For this review, use the dimensioned drawing (mm, ordinates from the lowest corner) and the shaded views. A direction names the side the tool comes from. Coordinates: 2 decimals unless noted, no trailing zeros. Write each loop counter-clockwise with the first axis right and the second up, starting at its lowest first coordinate (ties: lowest second). Pieces come first, ordered by that corner, then holes. Notation, with made-up numbers: (77.5, 28.25) - (99.5, 28.25) arc R17 ccw to (99.5, 43.25) - close; hole circle Ø5 at (39.25, 75). An arc over 180 degrees is marked (long way). One line per item, written item: value.
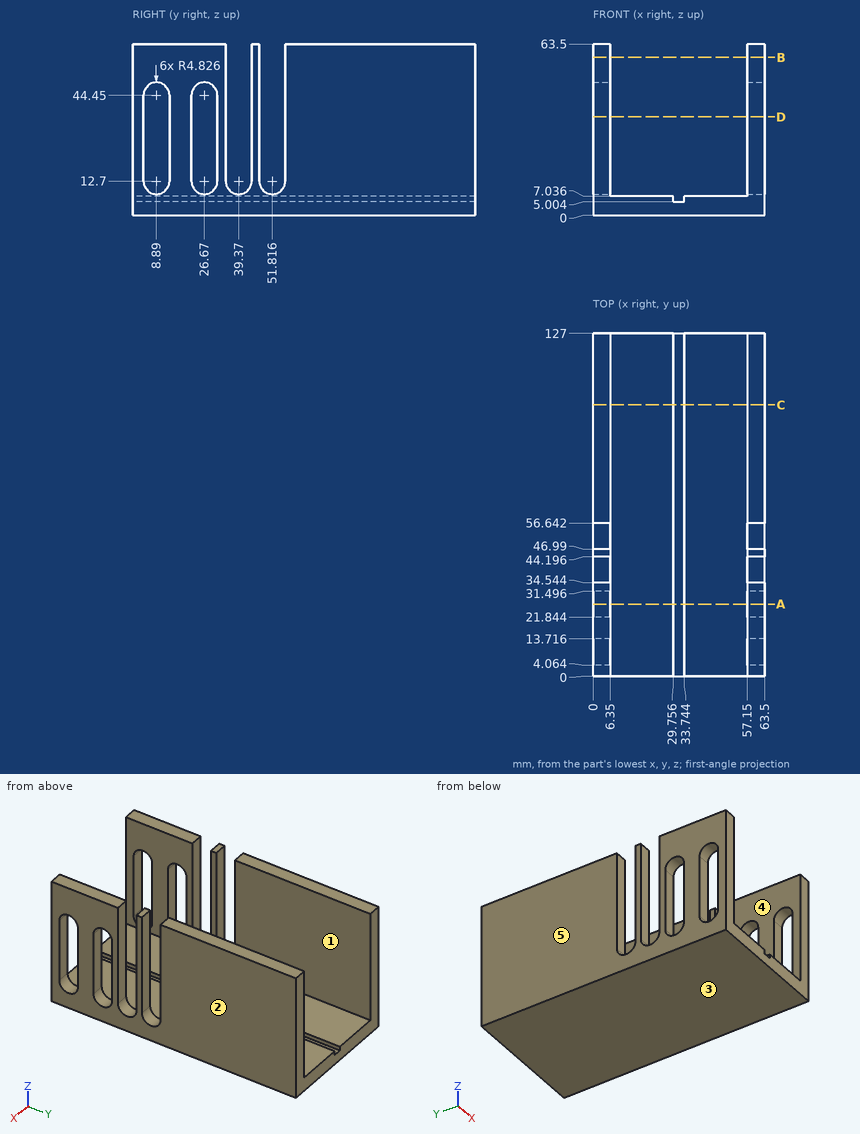
1. Consider section C-C, the plane y = 100.5. Write out the cut boundary in (x, z), then the cut area to 3 significant figures.
Answer block:
outline: (0, 0) - (63.5, 0) - (63.5, 63.5) - (57.15, 63.5) - (57.15, 7.04) - (33.74, 7.04) - (33.74, 5) - (29.76, 5) - (29.76, 7.04) - (6.35, 7.04) - (6.35, 63.5) - (0, 63.5) - close
area: 1,160 mm^2
2. Mouldability with a two-part tool opening along X and no side actions: class the marked faces 1, 2 and 3 as released by +X, released by -X, zero draft, split by the parting line, or undercut.
Answer block:
face 1: undercut
face 2: released by +X
face 3: zero draft
3. Insertion check: pin 1 Ø5 at (x, y) = (23.5, 37) entering from +Z. The pin has a flat end and moves straight along its axis. Give the tip position at first contact, or say it passes through.
Answer block:
pin 1: stops at z = 7.04
4. Consider section B-B, the plane z = 58.5. Write out the cut boundary in (x, y), then the cut area to 3 significant figures.
Answer block:
outline: (0, 0) - (6.35, 0) - (6.35, 34.54) - (0, 34.54) - close; (0, 44.2) - (6.35, 44.2) - (6.35, 46.99) - (0, 46.99) - close; (0, 56.64) - (6.35, 56.64) - (6.35, 127) - (0, 127) - close; (57.15, 0) - (63.5, 0) - (63.5, 34.54) - (57.15, 34.54) - close; (57.15, 44.2) - (63.5, 44.2) - (63.5, 46.99) - (57.15, 46.99) - close; (57.15, 56.64) - (63.5, 56.64) - (63.5, 127) - (57.15, 127) - close
area: 1,370 mm^2
5. Wall thickness on line 1 along Y through (x, z) = (6, 58.5); line 2 along X through (y, z) = (114.5, 24.5); line 3 along Y through (x, z) = (5, 23): over which ranges is each line inside the solid? List them lowest first.
Answer block:
line 1: y = 0 to 34.54, 44.2 to 46.99, 56.64 to 127
line 2: x = 0 to 6.35, 57.15 to 63.5
line 3: y = 0 to 4.06, 13.72 to 21.84, 31.5 to 34.54, 44.2 to 46.99, 56.64 to 127
6. Consider section D-D, the plane z = 36.5. Give the number of separate pieces and of enclosed holes in the cut face, then the cut area to 3 significant figures.
Answer block:
separate pieces: 10
enclosed holes: 0
area: 1,120 mm^2
7. Consider section A-A, the plane y = 26.67. Write out the cut boundary in (x, z).
Answer block:
outline: (0, 0) - (63.5, 0) - (63.5, 7.87) - (57.15, 7.87) - (57.15, 7.04) - (33.74, 7.04) - (33.74, 5) - (29.76, 5) - (29.76, 7.04) - (6.35, 7.04) - (6.35, 7.87) - (0, 7.87) - close; (0, 49.28) - (6.35, 49.28) - (6.35, 63.5) - (0, 63.5) - close; (57.15, 49.28) - (63.5, 49.28) - (63.5, 63.5) - (57.15, 63.5) - close
8. For the marked faces 4 and 5, list the 3-axis set-ups (+Z, -Z, +X, -X, +Y, -Y) from which the entire face can be reached by the end or side of a thin tool; tool diameter is ignored.
Answer block:
face 4: +Z, +Y, -Y
face 5: +Z, -Z, -X, +Y, -Y
